from build123d import *

# Parameters (mm, degrees)
SKETCH_2_W          = 40
SKETCH_2_H          = 41
SKETCH_2_R          = 1.6
EXTRUDE_1_DEPTH     = 40.2
SKETCH_3_W          = 40
SKETCH_3_H          = 39
CUT_EXTRUDE_1_DEPTH = 38.2
CUT_EXTRUDE_2_DEPTH = 60.604020905
SKETCH_5_R          = 1.6
CUT_EXTRUDE_3_DEPTH = 60.604020905
FILLET_1_R          = 3


with BuildPart() as part:
    # 草图2 → 凸台-拉伸1 (new body)
    with BuildSketch(Plane.XY):
        with Locations((0.386252919, 6.049930002)):
            Rectangle(SKETCH_2_W, SKETCH_2_H)
        with Locations(Location((-14.613747081, -6.450069998, 0), (0, 0, 180))):
            Circle(SKETCH_2_R, mode=Mode.SUBTRACT)
        with Locations(Location((15.386252919, -6.450069998, 0), (0, 0, 180))):
            Circle(SKETCH_2_R, mode=Mode.SUBTRACT)
        with Locations(Location((-14.613747081, 17.549930002, 0), (0, 0, 180))):
            Circle(SKETCH_2_R, mode=Mode.SUBTRACT)
        with Locations(Location((15.386252919, 17.549930002, 0), (0, 0, 180))):
            Circle(SKETCH_2_R, mode=Mode.SUBTRACT)
    extrude(amount=EXTRUDE_1_DEPTH)

    # 草图3 → 切除-拉伸1 (cut)
    with BuildSketch(Plane.XY.offset(40.2)):
        with Locations((0.386252919, 5.049930002)):
            Rectangle(SKETCH_3_W, SKETCH_3_H)
    extrude(amount=-CUT_EXTRUDE_1_DEPTH, mode=Mode.SUBTRACT)

    # 草图4 → 切除-拉伸2 (cut, through all)
    with BuildSketch(Plane.XZ.offset(-24.549930002)):
        with BuildLine():
            Line((-2.435094277, 40.2), (-19.613747081, 40.2))
            Line((-19.613747081, 40.2), (-19.613747081, 20.4))
            ThreePointArc((-19.613747081, 20.4), (-14.720483061, 33.50673598), (-2.435094277, 40.2))
        make_face()
        with BuildLine():
            Line((20.386252919, 40.2), (3.207600115, 40.2))
            ThreePointArc((3.207600115, 40.2), (15.492988899, 33.50673598), (20.386252919, 20.4))
            Line((20.386252919, 20.4), (20.386252919, 40.2))
        make_face()
    extrude(amount=-CUT_EXTRUDE_2_DEPTH, mode=Mode.SUBTRACT)

    # 草图5 → 切除-拉伸3 (cut, through all)
    with BuildSketch(Plane.XZ.offset(-24.549930002)):
        with Locations(Location((-15.113747081, 20.4, 0), (0, 0, 270))):
            Circle(SKETCH_5_R)
        with Locations(Location((15.886252919, 20.4, 0), (0, 0, 270))):
            Circle(SKETCH_5_R)
        with Locations(Location((-7.363747081, 33.823393759, 0), (0, 0, 270))):
            Circle(SKETCH_5_R)
        with Locations(Location((8.136252919, 33.823393759, 0), (0, 0, 270))):
            Circle(SKETCH_5_R)
        with Locations(Location((-7.363747081, 6.976606241, 0), (0, 0, 270))):
            Circle(SKETCH_5_R)
        with Locations(Location((8.136252919, 6.976606241, 0), (0, 0, 270))):
            Circle(SKETCH_5_R)
        with BuildLine():
            Line((-5.613747081, 12.9), (-5.613747081, 27.9))
            ThreePointArc((-5.613747081, 27.9), (0.386252919, 33.9), (6.386252919, 27.9))
            Line((6.386252919, 27.9), (6.386252919, 12.9))
            ThreePointArc((6.386252919, 12.9), (0.386252919, 6.9), (-5.613747081, 12.9))
        make_face()
    extrude(amount=-CUT_EXTRUDE_3_DEPTH, mode=Mode.SUBTRACT)

    # 圆角1
    fillet_1_edges = [part.edges().sort_by_distance(p)[0] for p in [
        (20.386252919, -14.450069998, 1),
        (-19.613747081, -14.450069998, 1),
    ]]
    fillet(fillet_1_edges, radius=FILLET_1_R)


solid = part.part
Build history of the part. All positions in model axes, mm. A direction names the side the tool comes from. Coordinates: 2 decimals unless noted, no trailing zeros. Write each loop counter-clockwise with the first axis right and the second up, starting at its lowest first coordinate (ties: lowest second). Pieces come first, ordered by that corner, then holes. Notation, with made-up numbers: (59.25, 51) -> (73.25, 51) arc R21 ccw to (73.25, 90) -> close; hole circle Ø1 at (81.5, 42.25). An arc over 180 degrees is marked (long way). Use CSV: the item, a comma, the result in double quotes. Start each with the question number.
Q1. Drill centre lines: probe 1 along X at (y, z) = (25.95, 20.4); probe 2 along X at (y, z) = (25, 20); probe 3 along Y at (x, z) = (14.5, 13.5). Where is each one in solid material? Low to high.
Q2. Pull direction X, two halves, no side cores. Call faces 4 (the flat face through (0, 26, 40.2)), 5 (the flat face through (20.386, 10.3, 1.8)), 6 (the cylindrical face through (-14.032, 25.536, 21.579)): released by +X, released by -X, zero draft, split by the parting line, or undercut.
Q3. 3-axis set-ups, long thin cutter, end or side, ignore diameter. For faces 1 (the flat face through (9, 24.55, 17)), 2 (the flat face through (-5.614, 26, 20)), 3 (the flat face through (-9, 26.55, 20)): which of +Z, -Z, +X, -X, +Y, -Y reach the whole face in a straight line?
Q4. Cut at C-C, the plane x = -12. List the corners of the cut face in (y, z).
Q5. Cut at A-A, the plane z = 23. List the corners of the cut face in (x, y), then the cut area to 3 significant figures.
Q6. Flat gauge pins, fed straight in: pin 1 Ø12 at (x, y) = (16, -6) entering from +Z; pin 2 Ø4 at (x, z) = (-12.5, 13.5) entering from -Y; pin 3 Ø2 at (y, z) = (26, 23.5) entering from +X. Where does each tip first touch, or does it go through?
Q7. Cut at B-B, the plane y = 14.5. List the corners of the cut face in (x, z), then the cut area to 3 significant figures.
Checked values:
1,probe 1,"x = -19.61 to -16.71, -13.51 to -5.61, 6.39 to 14.29, 17.49 to 20.39"
1,probe 2,"x = -19.61 to -16.66, -13.56 to -5.61, 6.39 to 14.34, 17.44 to 20.39"
1,probe 3,"y = 24.55 to 26.55"
2,face 4,"zero draft"
2,face 5,"released by +X"
2,face 6,"undercut"
3,face 1,"+Z, +X, -X, -Y"
3,face 2,"+Y, -Y"
3,face 3,"+Z, -Z, +X, -X, +Y"
4,outline,"(-14.45, 0) -> (26.55, 0) -> (26.55, 36.1) -> (24.55, 36.1) -> (24.55, 2) -> (-14.45, 2) -> close"
5,outline,"(-19.44, 24.55) -> (-5.61, 24.55) -> (-5.61, 26.55) -> (-19.44, 26.55) -> close; (6.39, 24.55) -> (20.22, 24.55) -> (20.22, 26.55) -> (6.39, 26.55) -> close"
5,area,"55.3 mm²"
6,pin 1,"stops at z = 2"
6,pin 2,"stops at y = 24.55"
6,pin 3,"stops at x = 20.28"
7,outline,"(-19.61, 0) -> (20.39, 0) -> (20.39, 2) -> (-19.61, 2) -> close"
7,area,"80.0 mm²"
